Can you work these out from the model? Positions are in its coordinate system, mm. Face numbers are marked on the shaded views. A direction names the side the tool comes from. Round coordinates to 2 decimals unless told otherwise and drop trailing zeros. Order: outer loops, then holes, each group sorted by start corner. A loop starts at its lowest first (then second) coordinate and runs counter-clockwise, first axis right, second up. Notation, with made-up numbers: M 9.25,-10.75 L 63.25,-10.75 A35 ccw 63.25,22.25 Z; hole C -36.5,18.25 d11. An arc over 180 degrees is marked long. Answer as a JSON object with one key per item and string values. Group by question number.
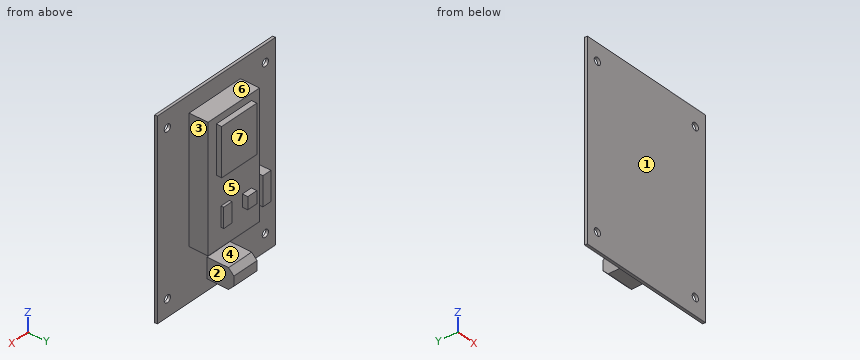
Autodesk Inventor part; units mm, degrees
ref_plane "YZ Plane" through (0, 0, 0) normal (1, 0, 0) x (0, 1, 0)
ref_plane "XZ Plane" through (0, 0, 0) normal (0, 1, 0) x (-1, 0, 0)
ref_plane "XY Plane" through (0, 0, 0) normal (0, 0, 1) x (1, 0, 0)
sketch "Esboço1" plane through (0, 0, 0) normal (0, 1, 0) x (-1, 0, 0)
  line L0 (-25.5, 35.75) -> (25.5, 35.75)
  line L1 (25.5, 35.75) -> (25.5, -35.75)
  line L2 (25.5, -35.75) -> (-25.5, -35.75)
  line L3 (-25.5, -35.75) -> (-25.5, 35.75)
  line L4 (-25.5, 35.75) -> (25.5, -35.75) construction
  line L5 (25.5, 35.75) -> (-25.5, -35.75) construction
  circle A0 centre (21.15, 29.4) radius 1.35
  circle A1 centre (-21.15, 29.4) radius 1.35
  line L6 (35.4001, 0) -> (-36.6047, 0)
  circle A2 centre (21.15, -29.4) radius 1.35
  circle A3 centre (-21.15, -29.4) radius 1.35
  point P0 (0, 0)
  dimension "d0" = 51
  dimension "d1" = 71.5
  dimension "d2" = 2.7
  dimension "d3" = 3
  dimension "d4" = 5
  dimension "d5" = 2.7
  dimension "d6" = 5
  dimension "d7" = 3
extrude "Extrusão1" add sketch "Esboço1" along normal blind 1
sketch "Esboço2" plane through (0, 1, 0) normal (0, 1, 0) x (1, 0, 0)
  line L0 (-25.5, 35.75) -> (-25.5, -35.75)
  line L1 (-25.5, -35.75) -> (25.5, -35.75)
  line L2 (25.5, 35.75) -> (-25.5, 35.75)
  line L3 (25.5, -35.75) -> (25.5, 35.75)
  line L4 (-10.4597, -29.5298) -> (11.731, -29.5298)
  line L5 (11.731, -29.5298) -> (11.731, 16.4696)
  line L6 (11.731, 16.4696) -> (-10.4597, 16.4696)
  line L7 (-10.4597, 16.4696) -> (-10.4597, -29.5298)
  line L8 (-15.4294, 1.4447) -> (-11.9622, 1.4447)
  line L9 (-11.9622, 1.4447) -> (-11.9622, 12.1933)
  line L10 (-11.9622, 12.1933) -> (-15.4294, 12.1933)
  line L11 (-15.4294, 12.1933) -> (-15.4294, 1.4447)
  line L12 (-5.9522, 24.0977) -> (4.0478, 24.0977)
  line L13 (4.0478, 24.0977) -> (4.0478, 31.5977)
  line L14 (4.0478, 31.5977) -> (-5.9522, 31.5977)
  line L15 (-5.9522, 31.5977) -> (-5.9522, 24.0977)
  point P0 (0, 0)
  dimension "d12" = 10
  dimension "d13" = 7.5
extrude "Extrusão2" add sketch "Esboço2" along normal blind 7 contours L7 L6 L5 L4 | L11 L10 L9 L8
extrude "Extrusão3" add sketch "Esboço2" along normal blind 10 contours L15 L14 L13 L12
chamfer "Chanfro1" distance 2 angle 45 2 edges at (-0.9522, 11, -24.0977) (-0.9522, 11, -31.5977)
sketch "Esboço3" plane through (0, 8, 0) normal (0, 1, 0) x (1, 0, 0)
  line L0 (-10.4597, 16.4696) -> (-10.4597, -29.5298)
  line L1 (-10.4597, -29.5298) -> (11.731, -29.5298)
  line L2 (11.731, 16.4696) -> (-10.4597, 16.4696)
  line L3 (11.731, -29.5298) -> (11.731, 16.4696)
  line L4 (-6.9899, -27.068) -> (8.1586, -27.068)
  line L5 (8.1586, -27.068) -> (8.1586, -9.4197)
  line L6 (8.1586, -9.4197) -> (-6.9899, -9.4197)
  line L7 (-6.9899, -9.4197) -> (-6.9899, -27.068)
  line L8 (-6.9899, 3.0291) -> (-3.1403, 3.0291)
  line L9 (-3.1403, 3.0291) -> (-3.1403, 7.5786)
  line L10 (-3.1403, 7.5786) -> (-6.9899, 7.5786)
  line L11 (-6.9899, 7.5786) -> (-6.9899, 3.0291)
  line L12 (2.5592, 2.2291) -> (6.1088, 2.2291)
  line L13 (6.1088, 2.2291) -> (6.1088, 9.5784)
  line L14 (6.1088, 9.5784) -> (2.5592, 9.5784)
  line L15 (2.5592, 9.5784) -> (2.5592, 2.2291)
  point P0 (0, 0)
extrude "Extrusão4" add sketch "Esboço3" along normal blind 2 contours L7 L6 L5 L4 | L11 L10 L9 L8
extrude "Extrusão5" add sketch "Esboço3" along normal blind 1 contours L15 L14 L13 L12
properties part number "PCB"
1) I need wall thicknesses on line 1 along Z through (x, y) = (-21.15, 0.2); line 2 along Y through (x, z) = (22.5, 33); line 3 along Y through (x, z) = (3, -5). Which ranges of each line are inside material? Lowest first, please.
2) If we section it at D-D on z = 15: Write out the boundary of the cut face in (x, y).
3) Which directions (+Z, -Z, +X, -X, +Y, -Y) give clear straight access to the entire face, cutting with the end or side of a thin tool? Please do the marked faces 1, 2 and 3.
4) We'd pull the mould along Z, two halves only. Please class the marked faces 4, 5, 6 and 7: +Z half, -Z half, draft (parallel to the pull), parting line (faces both ways), or undercut.
5) If we section it at A-A on y = 4: Write out the boundary of the cut face in (x, z).
6) For pin 1 (18 mm diameter, centred on x = 4, z = 14.5, fed in from +Y); pin 2 (4 mm diameter, centred on x = -12, y = 9, fed in from -Z); pin 3 (3.5 mm diameter, centred on y = 3, z = -2, fed in from +X); pin 4 (2 mm diameter, centred on y = 7.5, z = -22.5, fed in from -X), each with a flat end and sliding along its axis, tell me the tip position at first contact or that it passes through.
7) If we section it at C-C on x = -8: Write out the boundary of the cut face in (y, z), plus the area to 3 significant figures.
8) If we section it at B-B on x = 21.15: Write out the boundary of the cut face in (y, z), plus the area to 3 significant figures.
Findings:
{
 "1": {"line 1": "z = -35.75 to -30.75, -28.05 to 28.05, 30.75 to 35.75", "line 2": "y = 0 to 1", "line 3": "y = 0 to 9"},
 "2": {"outline": "M -25.5,0 L 25.5,0 L 25.5,1 L 11.73,1 L 11.73,8 L 8.16,8 L 8.16,10 L -6.99,10 L -6.99,8 L -10.46,8 L -10.46,1 L -25.5,1 Z"},
 "3": {"face 1": "+Z, -Z, +X, -X, -Y", "face 2": "-Z, +X, +Y", "face 3": "+Z, -Z, +X, +Y"},
 "4": {"face 4": "undercut", "face 5": "undercut", "face 6": "+Z half", "face 7": "draft"},
 "5": {"outline": "M -15.43,-12.19 L -11.96,-12.19 L -11.96,-1.44 L -15.43,-1.44 Z; M -10.46,-16.47 L 11.73,-16.47 L 11.73,29.53 L -10.46,29.53 Z; M -5.95,-31.6 L 4.05,-31.6 L 4.05,-24.1 L -5.95,-24.1 Z"},
 "6": {"pin 1": "stops at y = 10", "pin 2": "stops at z = -16.47", "pin 3": "stops at x = 11.73", "pin 4": "passes through"},
 "7": {"outline": "M 0,-35.75 L 1,-35.75 L 1,-16.47 L 8,-16.47 L 8,29.53 L 1,29.53 L 1,35.75 L 0,35.75 Z", "area": "393 mm^2"},
 "8": {"outline": "M 0,-35.75 L 1,-35.75 L 1,-30.75 L 0,-30.75 Z; M 0,-28.05 L 1,-28.05 L 1,28.05 L 0,28.05 Z; M 0,30.75 L 1,30.75 L 1,35.75 L 0,35.75 Z", "area": "66.1 mm^2"}
}
